Could you check a few things on this model? Use its own coordinates, in mm. Give positions to 0.01 mm unless a question says otherwise; leave off trailing zeros. Order: outer loops, then holes, each group sorted by start corner. A loop starts at its lowest first (then second) coordinate and runs counter-clockwise, first axis right, second up. Notation, with made-up numbers: (32, 20.5) - (70, 20.5) arc R12 cw to (70, 41.5) - close; hole circle Ø4 at (30, -28.5). An arc over 180 degrees is marked (long way). Put each result on its own line as item: value.
Autodesk Inventor part; units mm, degrees
ref_plane "YZ Plane" through (0, 0, 0) normal (1, 0, 0) x (0, 1, 0)
ref_plane "XZ Plane" through (0, 0, 0) normal (0, 1, 0) x (-1, 0, 0)
ref_plane "XY Plane" through (0, 0, 0) normal (0, 0, 1) x (1, 0, 0)
sketch "Szkic1" plane through (0, 0, 0) normal (0, 1, 0) x (-1, 0, 0)
  line L0 (34.6, 10.4209) -> (34.6, 8.4209)
  line L1 (34.6, 8.4209) -> (50, 8.4209)
  line L2 (50, 8.4209) -> (50, 10.4209)
  line L3 (50, 10.4209) -> (34.6, 10.4209)
  line L4 (0, 0) -> (0, 76.2035)
  dimension "d0" = 15.4
  dimension "d1" = 2
  dimension "d2" = 34.6
revolve "Obrót1" add sketch "Szkic1" angle 360 about axis through (0, 0, 0) along (0, 0, 1)
sketch "Szkic5" plane through (0, 0, 10.4209) normal (0, 0, 1) x (1, 0, 0)
  circle A0 centre (0, 40) radius 3
  circle A1 centre (40, 0) radius 3
  circle A2 centre (0, -40) radius 3
  circle A3 centre (-40, 0) radius 3
  point P0 (0, 0)
  dimension "d16" = 6
  dimension "d17" = 6
  dimension "d18" = 6
  dimension "d19" = 6
extrude "Wyciągnięcie proste3" cut sketch "Szkic5" against normal blind 2
properties part number "uszczelka" material "Poliwęglan dymiony"
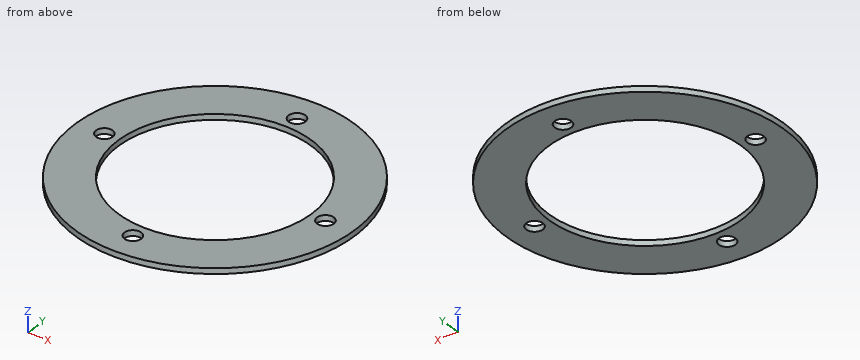
1) Suppose I cut it at A-A, the plane x = 0. List the corners of the cut face in (y, z) for me.
Filled in:
outline: (-50, 8.42) - (-43, 8.42) - (-43, 10.42) - (-50, 10.42) - close; (-37, 8.42) - (-34.6, 8.42) - (-34.6, 10.42) - (-37, 10.42) - close; (34.6, 8.42) - (37, 8.42) - (37, 10.42) - (34.6, 10.42) - close; (43, 8.42) - (50, 8.42) - (50, 10.42) - (43, 10.42) - close
2) Suppose I cut it at D-D, the plane z = 9.8. List the corners of the cut face in (x, y) for me, and give its area (3 significant figures).
Filled in:
outline: circle Ø100 at (0, 0); hole circle Ø6 at (-40, 0); hole circle Ø69.2 at (0, 0); hole circle Ø6 at (0, -40); hole circle Ø6 at (0, 40); hole circle Ø6 at (40, 0)
area: 3,980 mm^2
3) I'm going to push a flat-ended pin straight in: pin 1 (1 mm diameter, centred on x = -14, z = 9, fed in from +Y). Where does the tip first touch, or does it pass through?
Filled in:
pin 1: stops at y = 48.14
4) If I drill on line 1 (Y direction, x = 0, z = 8.8); line 2 (Y direction, x = -17.5, z = 10); line 3 (Y direction, x = -39.5, z = 9.2), over which ranges is the centre line in solid material (lowest first)? Write a range as [from, to].
Filled in:
line 1: y = [-50, -43], [-37, -34.6], [34.6, 37], [43, 50]
line 2: y = [-46.84, -29.85], [29.85, 46.84]
line 3: y = [-30.66, -2.96], [2.96, 30.66]
5) Suppose I cut it at B-B, the plane y = 40. List the corners of the cut face in (x, z) for me.
Filled in:
outline: (-30, 8.42) - (-3, 8.42) - (-3, 10.42) - (-30, 10.42) - close; (3, 8.42) - (30, 8.42) - (30, 10.42) - (3, 10.42) - close
